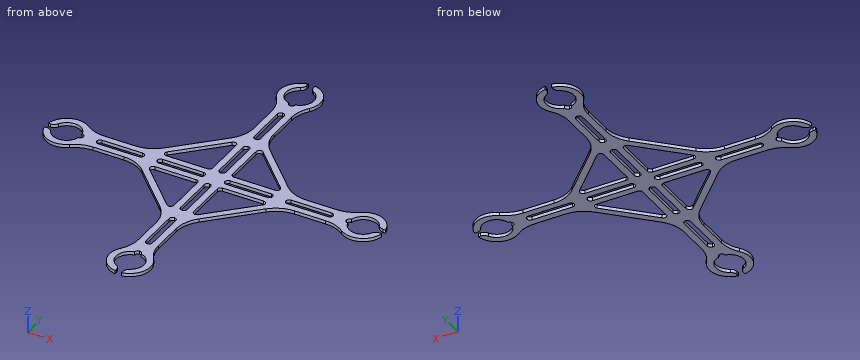
```python
from build123d import *

# Parameters (mm, degrees)
PAD_DEPTH   = 1
FILLET_R    = 2
FILLET001_R = 10
FILLET002_R = 1


with BuildPart() as fillet002:
    # Sketch → Pad (new body)
    with BuildSketch(Plane.XY):
        with BuildLine():
            ThreePointArc((-16.5, 1), (-17.207107, 0.707107), (-17.5, 0))
            Line((-17.5, 0), (-21.5, 0))
            ThreePointArc((-21.5, 0), (-21.792893, 0.707107), (-22.5, 1))
            Line((-22.5, 1), (-34.869322, 1))
            ThreePointArc((-34.869322, 1), (-35.576429, 0.707107), (-35.869322, 0))
            Line((-39.869322, 0), (-35.869322, 0))
            ThreePointArc((-39.869322, 0), (-40.162215, 0.707107), (-40.869322, 1))
            ThreePointArc((-40.869322, 1), (-45, 4.25), (-49.130678, 1))
            Line((-49.130678, 1), (-51.169481, 1))
            ThreePointArc((-39.517072, 3), (-46.057279, 6.159924), (-51.169481, 1))
            Line((-39.517072, 3), (-21.748737, 3))
            Line((-21.748737, 3), (-3, 21.748737))
            Line((-3, 21.748737), (-3, 39.517072))
            ThreePointArc((-1, 51.169481), (-6.159924, 46.057279), (-3, 39.517072))
            Line((-1, 51.169481), (-1, 49.130678))
            ThreePointArc((-1, 49.130678), (-4.25, 45), (-1, 40.869322))
            ThreePointArc((-1, 40.869322), (-0.707107, 40.162215), (0, 39.869322))
            Line((0, 39.869322), (0, 35.869322))
            ThreePointArc((0, 35.869322), (-0.707107, 35.576429), (-1, 34.869322))
            Line((-1, 22.5), (-1, 34.869322))
            ThreePointArc((-1, 22.5), (-0.707107, 21.792893), (0, 21.5))
            Line((0, 21.5), (0, 17.5))
            ThreePointArc((0, 17.5), (-0.707107, 17.207107), (-1, 16.5))
            Line((-1, 4), (-1, 16.5))
            ThreePointArc((-1, 4), (-0.707107, 3.292893), (0, 3))
            Line((0, 3), (0, 0))
            Line((0, 0), (-3, 0))
            ThreePointArc((-3, 0), (-3.292893, 0.707107), (-4, 1))
            Line((-16.5, 1), (-4, 1))
        make_face()
        Polygon((-3, 3), (-18.92031, 3), (-3, 18.92031), align=None, mode=Mode.SUBTRACT)
    extrude(amount=PAD_DEPTH)

    # Fillet
    fillet_edges = [fillet002.edges().sort_by_distance(p)[0] for p in [
        (-49.130678, 1, 0.5),
        (-1, 49.130678, 0.5),
    ]]
    fillet(fillet_edges, radius=FILLET_R)

    # Fillet001
    fillet001_edges = [fillet002.edges().sort_by_distance(p)[0] for p in [
        (-3, 39.517072, 0.5),
        (-3, 21.748737, 0.5),
        (-21.748737, 3, 0.5),
        (-39.517072, 3, 0.5),
    ]]
    fillet(fillet001_edges, radius=FILLET001_R)

    # Fillet002
    fillet002_edges = [fillet002.edges().sort_by_distance(p)[0] for p in [
        (-3, 3, 0.5),
        (-3, 18.92031, 0.5),
        (-18.92031, 3, 0.5),
    ]]
    fillet(fillet002_edges, radius=FILLET002_R)


with BuildPart() as part_mirroring:
    # Part__Mirroring: instance of Fillet002
    add(fillet002.part.mirror(Plane(origin=(0, 0, 0), x_dir=(1, 0, 0), z_dir=(0, 1, 0))))


with BuildPart() as part_mirroring001:
    # Part__Mirroring001: instance of Part__Mirroring
    add(part_mirroring.part.mirror(Plane(origin=(0, 0, 0), x_dir=(0, -1, 0), z_dir=(1, 0, 0))))


with BuildPart() as fusion:
    # Part__Mirroring002: instance of Part__Mirroring001
    add(part_mirroring001.part.mirror(Plane(origin=(0, 0, 0), x_dir=(1, 0, 0), z_dir=(0, 1, 0))))

    # Fusion: union Part__Mirroring001, Fillet002, Part__Mirroring
    add(part_mirroring001.part)
    add(fillet002.part)
    add(part_mirroring.part)


solid = fusion.part
```
Can you work these out from the model? Positions are in its coordinate system, mm. Round coordinates to 2 decimals unless told otherwise and drop trailing zeros. Loops run counter-clockwise (first coordinate to the right, second up) from the corner with the lowest first, then second, coordinate; pieces in that order, holes last. Notation, with made-up numbers: (83.5, 43) -> (137.5, 43) arc R13 cw to (137.5, 58) -> close; hole circle Ø10 at (-21, -2.75). An arc over 180 degrees is marked (long way). Answer in a Markdown table with one row per item.
Item 1: If I drill on probe 1 along X at (y, z) = (32, 0.35); probe 2 along Y at (x, z) = (0.5, 0.4); probe 3 along X at (y, z) = (12, 0.55), over which ranges is the centre line in solid material (lowest first)?
Answer block:
| item | result |
|---|---|
| probe 1 | -3 to -1, 1 to 3 |
| probe 2 | -40 to -35.74, -21.63 to -17.37, -3.13 to 3.13, 17.37 to 21.63, 35.74 to 40 |
| probe 3 | -12.75 to -9.92, -3 to -1, 1 to 3, 9.92 to 12.75 |
Item 2: Will these pins go through, and if not, where does the flat tip stop? P1, Ø0.5, axis at y = 12.5, z = 0.5, coming from the +X side; P2, Ø0.5, axis at y = -31, z = 0.5, coming from the -X side; P3, Ø0.5, axis at x = -50.5, z = 0.5, coming from the -Y side.
Answer block:
| item | result |
|---|---|
| P1 | x = 12.5 |
| P2 | x = -3 |
| P3 | y = -3.39 |
Item 3: Suppose I cut it at D-D, the plane y = -10.5. List the corners of the cut face in (x, z) for me, plus the area to 3 significant figures.
Answer block:
| item | result |
|---|---|
| outline | (-14.25, 0) -> (-11.42, 0) -> (-11.42, 1) -> (-14.25, 1) -> close; (-3, 0) -> (-1, 0) -> (-1, 1) -> (-3, 1) -> close; (1, 0) -> (3, 0) -> (3, 1) -> (1, 1) -> close; (11.42, 0) -> (14.25, 0) -> (14.25, 1) -> (11.42, 1) -> close |
| area | 9.66 mm² |
Item 4: Suppose I cut it at A-A, the plane x = -32. List the corners of the cut face in (y, z) for me, plus the area to 3 significant figures.
Answer block:
| item | result |
|---|---|
| outline | (-3, 0) -> (-1, 0) -> (-1, 1) -> (-3, 1) -> close; (1, 0) -> (3, 0) -> (3, 1) -> (1, 1) -> close |
| area | 4.00 mm² |
Item 5: Suppose I cut it at B-B, the plane y = 44. List the corners of the cut face in (x, z) for me, plus the area to 3 significant figures.
Answer block:
| item | result |
|---|---|
| outline | (-6.17, 0) -> (-4.13, 0) -> (-4.13, 1) -> (-6.17, 1) -> close; (4.13, 0) -> (6.17, 0) -> (6.17, 1) -> (4.13, 1) -> close |
| area | 4.08 mm² |
Item 6: Suppose I cut it at C-C, the plane x = 14. List the corners of the cut face in (y, z) for me.
Answer block:
| item | result |
|---|---|
| outline | (-10.75, 0) -> (-7.92, 0) -> (-7.92, 1) -> (-10.75, 1) -> close; (-3, 0) -> (-1, 0) -> (-1, 1) -> (-3, 1) -> close; (1, 0) -> (3, 0) -> (3, 1) -> (1, 1) -> close; (7.92, 0) -> (10.75, 0) -> (10.75, 1) -> (7.92, 1) -> close |
